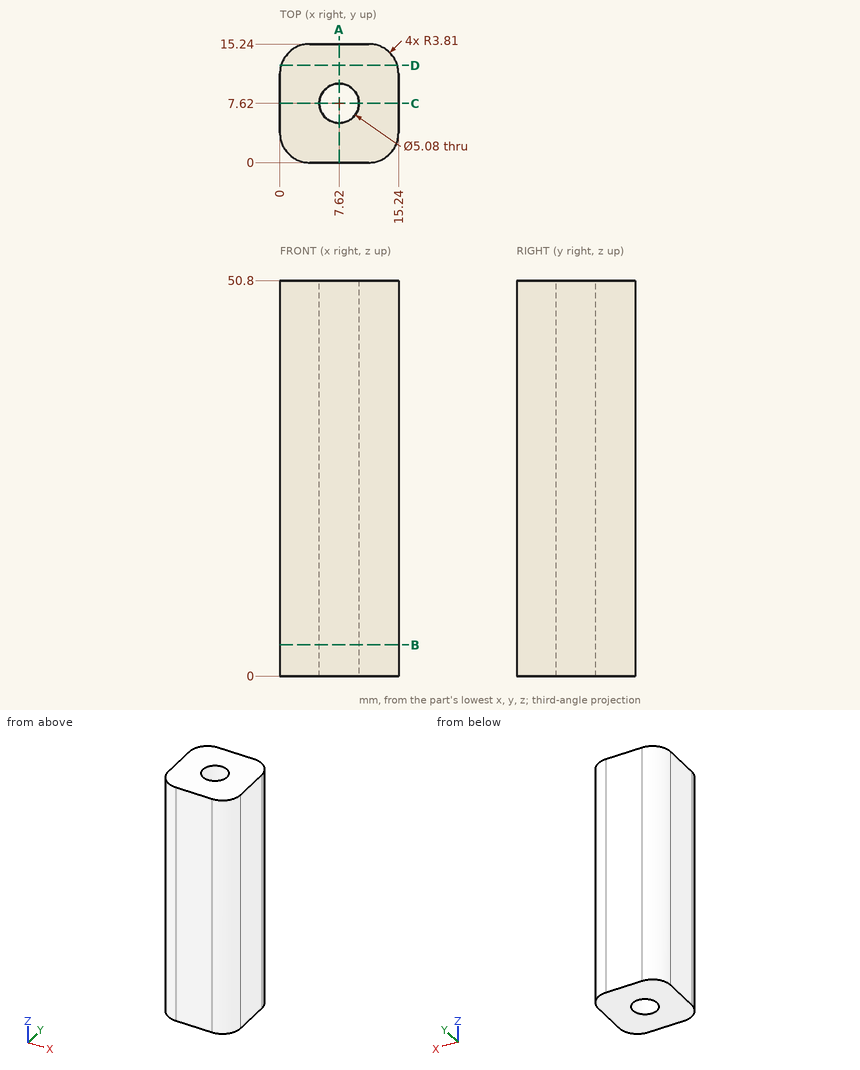
Answer from the drawing. Dimensions are ordinates in mm from the lowest x, y and z of the part. Coordinates: 2 decimals unless noted, no trailing zeros. Loops run counter-clockwise (first coordinate to the right, second up) from the corner with the lowest first, then second, coordinate; pieces in that order, holes last.
Q1. Consider probe 1 along X at (y, z) = (7.62, 35.5); probe 2 along Y at (x, z) = (7, 47.5). Determine where each line is inside the solid, lowest interval first.
Q2. The part is cut by section B-B on z = 4. Write down the section's boundary in (x, y), and give its area (3 significant figures).
Q3. The part is cut by section D-D on y = 12.5. Write down the section's boundary in (x, z), and give its area (3 significant figures).
Q4. The part is cut by section A-A on x = 7.62. Write down the section's boundary in (y, z), and give its area (3 significant figures).
Results below:
1. probe 1: x = 0 to 5.08, 10.16 to 15.24
1. probe 2: y = 0 to 5.16, 10.08 to 15.24
2. outline: (0, 3.81) arc R3.81 ccw to (3.81, 0) - (11.43, 0) arc R3.81 ccw to (15.24, 3.81) - (15.24, 11.43) arc R3.81 ccw to (11.43, 15.24) - (3.81, 15.24) arc R3.81 ccw to (0, 11.43) - close; hole circle Ø5.08 at (7.62, 7.62)
2. area: 200 mm2
3. outline: (0.15, 0) - (15.09, 0) - (15.09, 50.8) - (0.15, 50.8) - close
3. area: 759 mm2
4. outline: (0, 0) - (5.08, 0) - (5.08, 50.8) - (0, 50.8) - close; (10.16, 0) - (15.24, 0) - (15.24, 50.8) - (10.16, 50.8) - close
4. area: 516 mm2
